Part model, mm, in its own coordinate system. A direction names the side the tool comes from. Round coordinates to 2 decimals unless told otherwise and drop trailing zeros. Loops run counter-clockwise (first coordinate to the right, second up) from the corner with the lowest first, then second, coordinate; pieces in that order, holes last.
(1) Probe probe 1 along Z at (x, y) = (245, 119); probe 2 along Z at (x, y) = (637, 768); probe 3 along Y at (x, z) = (-230, -98.5). List the from-to ranges inside material, lowest first.
(2) Cut at D-D on y = 497. List the corners of the cut face in (x, z).
(3) Cut at B-B on y = 311.5. List the corners of the cut face in (x, z).
(4) Cut at C-C on x = 243.5. List the corners of the cut face in (y, z), then the cut area to 3 significant figures.
(5) Mould opens along X. For faces 1 (the face through (-196.86, 253.3, 262.66)), 2 (the face through (-9, 400, 0)), 3 (the face through (460.158, 570.173, 3.131)) say: +X half, -X half, draft (parallel to the pull), parting line (faces both ways), or undercut.
(6) Tool access for faces 4 (the face through (809.92, 861.88, 3.13)), 5 (the face through (4.795, 191.805, -149.89)), 6 (the face through (4.52, 187.62, 155.34)), 7 (the face through (-100.18, 424.13, 3.13)), 8 (the face through (-9, 292, 6.35)): list every direction of +Z, -Z, +X, -X, +Y, -Y with a clear straight run to the whole face (end or side of a thin tool).
(7) Cut at A-A on y = 617. List the corners of the cut face in (x, z).
from build123d import *

# Parameters (mm, degrees)
BOSS_EXTRUDE1_DEPTH = 6.35
BOSS_EXTRUDE2_DEPTH = 3.175


with BuildPart() as part:
    # Sketch1 → Boss-Extrude1 (new body)
    with BuildSketch(Plane.XY):
        Polygon((-304.8, 0), (304.8, 0), (690.659261151, 827.477855881), (907.061590086, 798.54952059), (710.019622074, 927.013433042), (203.2, 203.2), (0, 638.963806248), (-203.2, 203.2), (-791.008562204, 1042.677626458), align=None)
    extrude(amount=BOSS_EXTRUDE1_DEPTH)

    # Sketch2 → Boss-Extrude2 (add, symmetric)
    with BuildSketch(Plane(origin=(0, 76.2, 43.994090512), x_dir=(1, 0, 0), z_dir=(0, 0.866025403784438, 0.500000000000001))):
        Polygon((-352.176858069, 50.8), (-40.026997385, 660.4), (352.176858069, 50.8), align=None)
    boss_extrude2 = extrude(amount=BOSS_EXTRUDE2_DEPTH, both=True)

    # Mirror1: Boss-Extrude2 across plane
    add(boss_extrude2.mirror(Plane.XY))


solid = part.part
Final values:
1. probe 1: z = -36.49 to -23.79, 0 to 6.35, 23.79 to 36.49
1. probe 2: z = 0 to 6.35
1. probe 3: y = 154.8 to 162.14
2. outline: (-536.55, 0) - (-408.92, 0) - (-408.92, 6.35) - (-536.55, 6.35) - close; (-66.2, 0) - (66.2, 0) - (66.2, 6.35) - (-66.2, 6.35) - close; (408.92, 0) - (536.55, 0) - (536.55, 6.35) - (408.92, 6.35) - close
3. outline: (-450.05, 0) - (-279.03, 0) - (-279.03, 6.35) - (-450.05, 6.35) - close; (-152.7, 0) - (152.7, 0) - (152.7, 6.35) - (-152.7, 6.35) - close; (-140.03, -357.21) - (-134.4, -369.91) - (78.55, -369.91) - (85.62, -357.21) - close; (-140.03, 357.21) - (85.62, 357.21) - (78.55, 369.91) - (-134.4, 369.91) - close; (279.03, 0) - (450.05, 0) - (450.05, 6.35) - (279.03, 6.35) - close
4. outline: (0, 0) - (101.6, 0) - (98.85, -1.59) - (183.31, -147.87) - (188.81, -144.7) - (105.27, 0) - (260.75, 0) - (260.75, 6.35) - (108.93, 6.35) - (188.81, 144.7) - (183.31, 147.87) - (101.6, 6.35) - (0, 6.35) - close
4. area: 3,750 mm2
5. face 1: -X half
5. face 2: draft
5. face 3: undercut
6. face 4: +Z, -Z, +X, +Y
6. face 5: +X, -X, +Y
6. face 6: +Z, +X, -X, -Y
6. face 7: +Y
6. face 8: +X, -X
7. outline: (-592.51, 0) - (-492.95, 0) - (-492.95, 6.35) - (-592.51, 6.35) - close; (-10.24, 0) - (10.24, 0) - (10.24, 6.35) - (-10.24, 6.35) - close; (492.95, 0) - (592.51, 0) - (592.51, 6.35) - (492.95, 6.35) - close
